Here's the drawing with two shaded views (mm, measured from the low corner). I have some questions. A direction names the side the tool comes from. Round coordinates to 2 decimals unless told otherwise and drop trailing zeros. Loops run counter-clockwise (first coordinate to the right, second up) from the corner with the lowest first, then second, coordinate; pieces in that order, holes last.
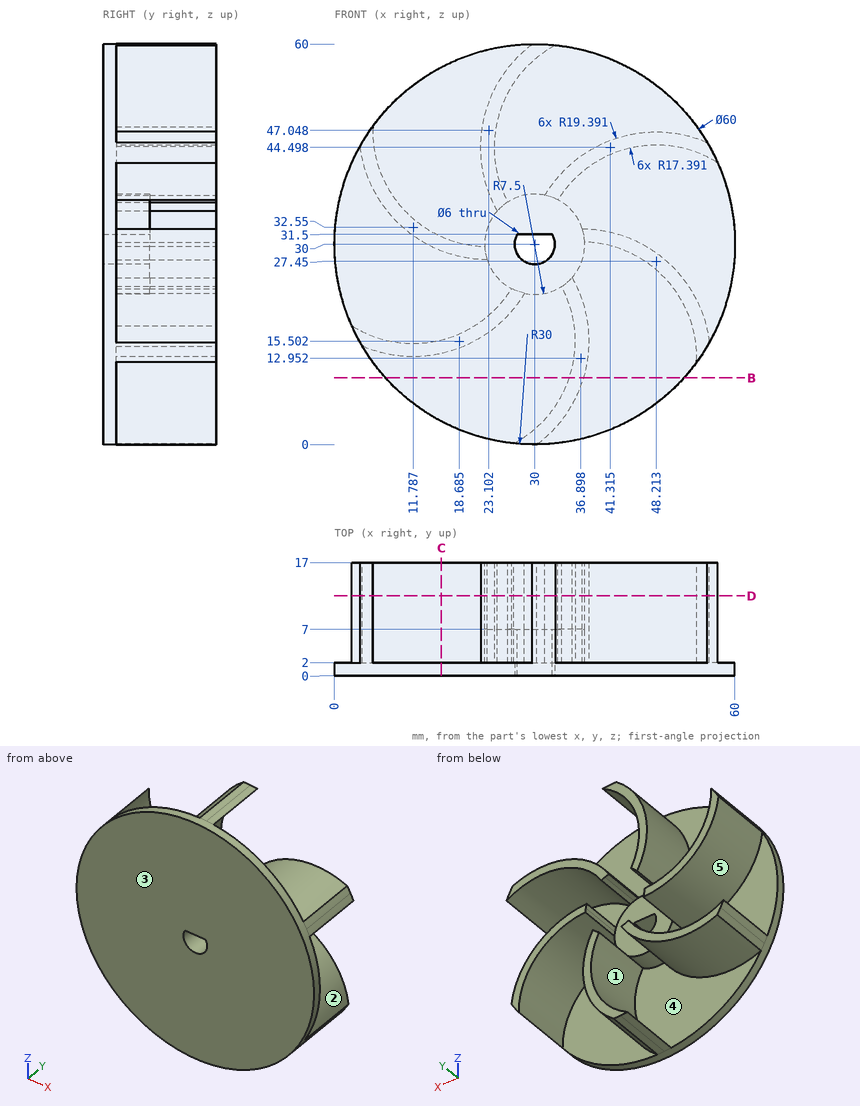
(1) If we section it at B-B, the plane z = 10: List the corners of the cut face in (x, y) for me, then the cut area to 3 significant figures.
Worked answers:
outline: (7.64, 0) - (52.36, 0) - (52.36, 2) - (37.28, 2) - (37.28, 17) - (35.18, 17) - (35.18, 2) - (7.64, 2) - close
area: 121 mm2
(2) If we section it at C-C, the plane x = 16: List the corners of the cut face in (y, z) for me (1 decimal).
Worked answers:
outline: (0, 3.5) - (2, 3.5) - (2, 13.6) - (17, 13.6) - (17, 15.7) - (2, 15.7) - (2, 29) - (17, 29) - (17, 31.2) - (2, 31.2) - (2, 56.5) - (0, 56.5) - close
(3) For the marked faces 4 and 5, which set-ups out of +Z, -Z, +X, -X, +Y, -Y let a thin tool reach every point of the face, with its end or its side?
Worked answers:
face 4: +Y
face 5: -X, +Y
(4) If I drill on line 1 (Z direction, x = 32, y = 7.25) (1 decimal); line 2 (Z direction, x = 30, y = 2.25) (1 decimal); line 3 (X direction, y = 4, z = 19) (1 decimal), over which ranges is the centre line in solid material (lowest first)?
Worked answers:
line 1: z = 1.4 to 4.3, 37.2 to 38.1, 59.2 to 59.9
line 2: z = 0 to 2.3, 22.5 to 27, 31.5 to 37.5, 57.7 to 60
line 3: x = 22.7 to 25.7, 35.7 to 37.8, 53.2 to 55.3
(5) If we section it at D-D, the plane y = 12: State how many separate pieces and enclosed holes the cut face has.
Worked answers:
separate pieces: 6
enclosed holes: 0
(6) Will these pins go through, and if not, where does the flat tip stop? P1, Ø5, axis at x = 35, y = 11.5, coming from the -Z side (1 decimal); P2, Ø5, axis at x = 30, z = 30, coming from the +Y side; P3, Ø19, axis at x = 43, z = 47, coming from the +Y side; P4, Ø6, axis at x = 7.5, y = 13, coming from the +Z side.
Worked answers:
P1: stops at z = 1.9
P2: stops at y = 7
P3: stops at y = 17
P4: stops at z = 47.62
(7) If we mould it in two halves opening along X, with no side actions, what happens to the marked faces 1, 2 and 3? For each: released by +X, released by -X, zero draft, split by the parting line, or undercut.
Worked answers:
face 1: undercut
face 2: released by +X
face 3: zero draft
